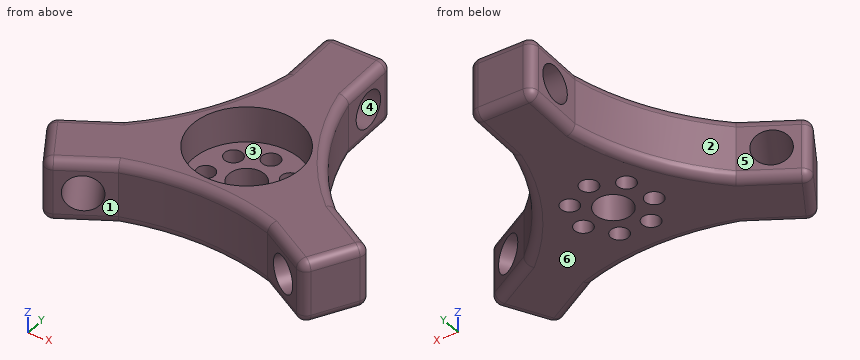
from build123d import *

# Parameters (mm, degrees)
SKETCH2_R           = 4
BOSS_EXTRUDE1_DEPTH = 14
SKETCH7_R           = 12.060749
CUT_EXTRUDE4_DEPTH  = 8
SKETCH8_R           = 2
CUT_EXTRUDE5_DEPTH  = 8
FILLET2_R           = 2
CUT_EXTRUDE6_REACH  = 53.745
SKETCH10_R          = 4
FILLET4_R           = 2
CIRPATTERN1_COUNT   = 3


with BuildPart() as part:
    # Sketch2 → Boss-Extrude1 (new body)
    with BuildSketch(Plane.XY):
        with BuildLine():
            Line((-7, 23), (-7, 37))
            Line((-7, 37), (7, 37))
            Line((7, 37), (7, 23))
            ThreePointArc((7, 23), (13.037466, 7.527184), (23.418584, -5.437822))
            Line((23.418584, -5.437822), (35.54294, -12.437822))
            Line((35.54294, -12.437822), (28.54294, -24.562178))
            Line((28.54294, -24.562178), (16.418584, -17.562178))
            ThreePointArc((16.418584, -17.562178), (0, -15.054369), (-16.418584, -17.562178))
            Line((-16.418584, -17.562178), (-28.54294, -24.562178))
            Line((-28.54294, -24.562178), (-35.54294, -12.437822))
            Line((-35.54294, -12.437822), (-23.418584, -5.437822))
            ThreePointArc((-23.418584, -5.437822), (-13.037466, 7.527184), (-7, 23))
        make_face()
        Circle(SKETCH2_R, mode=Mode.SUBTRACT)
    extrude(amount=BOSS_EXTRUDE1_DEPTH)

    # Sketch7 → Cut-Extrude4 (cut)
    with BuildSketch(Plane.XY.offset(14)):
        Circle(SKETCH7_R)
    extrude(amount=-CUT_EXTRUDE4_DEPTH, mode=Mode.SUBTRACT)

    # Sketch8 → Cut-Extrude5 (cut)
    with BuildSketch(Plane.XY.offset(6)):
        with Locations((0, 8)):
            Circle(SKETCH8_R)
        with Locations((6.254652, 4.987918)):
            Circle(SKETCH8_R)
        with Locations((7.799423, -1.780167)):
            Circle(SKETCH8_R)
        with Locations((3.47107, -7.207751)):
            Circle(SKETCH8_R)
        with Locations((-3.47107, -7.207751)):
            Circle(SKETCH8_R)
        with Locations((-7.799423, -1.780167)):
            Circle(SKETCH8_R)
        with Locations((-6.254652, 4.987918)):
            Circle(SKETCH8_R)
    extrude(amount=-CUT_EXTRUDE5_DEPTH, mode=Mode.SUBTRACT)

    # Fillet2
    fillet2_edges = [part.edges().sort_by_distance(p)[0] for p in [
        (32.04294, -18.5, 0),
        (-32.04294, -18.5, 0),
        (0, 37, 0),
        (-32.04294, -18.5, 14),
        (32.04294, -18.5, 14),
        (0, 37, 14),
    ]]
    fillet(fillet2_edges, radius=FILLET2_R)

    # Sketch10 → Cut-Extrude6 (cut, up to next)
    with BuildSketch(Plane(origin=(3.5, 6.062178, 0), x_dir=(0.866025403784439, -0.4999999999999995, 0), z_dir=(0.49999999999999944, 0.8660254037844389, 0)), mode=Mode.PRIVATE) as cut_extrude6_sk1:
        with Locations(Location((29.5, -7, 0), (0, 0, 180))):
            Circle(SKETCH10_R)
    cut_extrude6_tool1 = extrude(cut_extrude6_sk1.sketch, amount=-CUT_EXTRUDE6_REACH, mode=Mode.PRIVATE) & part.part
    cut_extrude6 = cut_extrude6_tool1.solids().sort_by_distance((29.047749, -8.687822, 7))[0]
    add(cut_extrude6, mode=Mode.SUBTRACT)

    # Fillet4
    fillet4_edges = [part.edges().sort_by_distance(p)[0] for p in [
        (7, 29, 0),
        (13.037466, 7.527184, 0),
        (-13.037466, 7.527184, 14),
        (21.614737, -20.562178, 0),
        (0, -15.054369, 0),
        (-28.614737, -8.437822, 0),
        (-13.037466, 7.527184, 0),
        (-28.614737, -8.437822, 14),
        (0, -15.054369, 14),
        (21.614737, -20.562178, 14),
        (13.037466, 7.527184, 14),
        (7, 29, 14),
        (-7, 37, 7),
        (7, 37, 7),
        (-7, 29, 0),
        (-7, 29, 14),
        (-7, 36.414214, 13.414214),
        (-7, 36.414214, 0.585786),
        (28.614737, -8.437822, 0),
        (-21.614737, -20.562178, 0),
        (7, 36.414214, 13.414214),
        (7, 36.414214, 0.585786),
        (-21.614737, -20.562178, 14),
        (28.614737, -8.437822, 14),
        (-28.54294, -24.562178, 7),
        (-35.54294, -12.437822, 7),
        (-28.035634, -24.269285, 13.414214),
        (-28.035634, -24.269285, 0.585786),
        (-35.035634, -12.144929, 13.414214),
        (-35.035634, -12.144929, 0.585786),
        (35.54294, -12.437822, 7),
        (28.54294, -24.562178, 7),
        (35.035634, -12.144929, 13.414214),
        (35.035634, -12.144929, 0.585786),
        (28.035634, -24.269285, 13.414214),
        (28.035634, -24.269285, 0.585786),
    ]]
    fillet(fillet4_edges, radius=FILLET4_R)

    # CirPattern1: Cut-Extrude6 ×3 about axis
    cirpattern1_axis = Axis((0, 0, 6), (0, 0, 1))
    for i in range(1, CIRPATTERN1_COUNT):
        add(cut_extrude6.rotate(cirpattern1_axis, i * 360 / CIRPATTERN1_COUNT), mode=Mode.SUBTRACT)


solid = part.part
Could you check a few things on this model? Use its own coordinates, in mm. Face numbers are marked on the shaded views. A direction names the side the tool comes from. Give positions to 0.01 mm unless a question says otherwise; leave off trailing zeros. Order: outer loops, then holes, each group sorted by start corner. A loop starts at its lowest first (then second) coordinate and runs counter-clockwise, first axis right, second up.
1. Suppose I cut it at A-A (y = 29.5). List the corners of the cut face in (x, z) for me.
2. For the marked faces 1, 2 and 3, which set-ups out of +Z, -Z, +X, -X, +Y, -Y let a thin tool reach every point of the face, with its end or its side?
3. Suppose I cut it at C-C (z = 7). Give the number of separate pieces and of enclosed holes in the cut face, plus the area to 3 significant figures.
4. I need wall thicknesses on L1, parallel to X at y = -13, z = 9; L2, parallel to Z at x = 1, y = 29.5; L3, parallel to X at y = 0, z = 3.8. Which ranges of each line are inside material? Lowest first, please.
5. Will these pins go through, and if not, where does the flat tip stop? P1, Ø6, axis at y = 12.5, z = 10.5, coming from the -X side; P2, Ø6.5, axis at x = 0, y = 0, coming from the -Z side; P3, Ø5, axis at x = -6.25, y = 4.99, coming from the +Z side; P4, Ø1.5, axis at x = -16.5, z = 6, coming from the -Y side.
6. We'd pull the mould along Z, two halves only. Please class the marked faces 4, 5 and 6: pulls with the +Z half, pulls with the -Z half, needs draft (parallel to the pull), parting line crosses it, or undercut.
7. Suppose I cut it at B-B (x = 0). List the corners of the cut face in (y, z) for me, plus the area to 3 significant figures.
Solved:
1. outline: (-7, 2) arc R2 ccw to (-5, 0) - (5, 0) arc R2 ccw to (7, 2) - (7, 3) - (-7, 3) - close; (-7, 11) - (7, 11) - (7, 12) arc R2 ccw to (5, 14) - (-5, 14) arc R2 ccw to (-7, 12) - close
2. face 1: +Z, -Z, -Y
2. face 2: +Z, -Z, -X, +Y
2. face 3: +Z
3. separate pieces: 4
3. enclosed holes: 1
3. area: 972 mm2
4. L1: x = -34.8 to -30.56, -22.56 to 22.56, 30.56 to 34.8
4. L2: z = 0 to 3, 11 to 14
4. L3: x = -18.26 to -8.71, -6.89 to -4, 4 to 6.89, 8.71 to 18.26
5. P1: stops at x = -11.95
5. P2: passes through
5. P3: stops at z = 6
5. P4: stops at y = -18.04
6. face 4: undercut
6. face 5: needs draft
6. face 6: pulls with the -Z half
7. outline: (-15.05, 2) arc R2 ccw to (-13.05, 0) - (-4, 0) - (-4, 6) - (-12.06, 6) - (-12.06, 14) - (-13.05, 14) arc R2 ccw to (-15.05, 12) - close; (4, 0) - (6, 0) - (6, 6) - (4, 6) - close; (10, 0) - (35, 0) arc R2 ccw to (37, 2) - (37, 12) arc R2 ccw to (35, 14) - (12.06, 14) - (12.06, 6) - (10, 6) - close; hole circle Ø8 at (29.5, 7)
7. area: 410 mm2
